Autodesk Inventor part; units mm, degrees
ref_plane "Work Plane1" through (36.5, 52.55, -8.75) normal (0, 0, 1) x (1, 0, 0)
ref_plane "YZ Plane" through (0, 0, 0) normal (1, 0, 0) x (0, 1, 0)
ref_plane "XZ Plane" through (0, 0, 0) normal (0, 1, 0) x (-1, 0, 0)
sketch "Sketch1" plane through (0, 0, 0) normal (0, 0, 1) x (1, 0, 0)
  line L0 (0, 44.8) -> (0, 9.25)
  line L1 (0, 44.8) -> (40, 44.8)
  line L2 (0, 9.25) -> (40, 9.25)
  line L3 (40, 9.25) -> (40, 44.8)
  line L4 (14.9707, 35.95) -> (34.6293, 35.95)
  line L5 (34.6293, 35.95) -> (34.6293, 40.05)
  line L6 (34.6293, 40.05) -> (14.9707, 40.05)
  line L7 (14.9707, 40.05) -> (14.9707, 35.95)
  line L8 (30.8793, 39.05) -> (28.5722, 39.05) construction
  line L9 (30.8793, 39.05) -> (30.8793, 36.95) construction
  line L10 (30.8793, 36.95) -> (28.5722, 36.95) construction
  line L11 (28.5722, 39.05) -> (28.5722, 36.95) construction
  line L12 (30.8793, 39.05) -> (30.8793, 40.05) construction
  line L13 (30.8793, 36.95) -> (30.8793, 35.95) construction
  line L14 (21.0278, 39.05) -> (18.7207, 39.05) construction
  line L15 (21.0278, 39.05) -> (21.0278, 36.95) construction
  line L16 (21.0278, 36.95) -> (18.7207, 36.95) construction
  line L17 (18.7207, 39.05) -> (18.7207, 36.95) construction
  line L18 (18.7207, 39.05) -> (14.9707, 39.05) construction
  line L19 (30.8793, 39.05) -> (34.6293, 39.05) construction
  line L20 (0, -9.25) -> (0, 9.25)
  line L21 (40, 27.025) -> (0, 27.025) construction
  line L22 (14.9707, 18.1) -> (34.6293, 18.1)
  line L23 (34.6293, 18.1) -> (34.6293, 14)
  line L24 (34.6293, 14) -> (14.9707, 14)
  line L25 (14.9707, 14) -> (14.9707, 18.1)
  line L26 (40, 9.25) -> (40, -9.25)
  line L27 (40, -9.25) -> (0, -9.25)
  line L28 (32.375, -9.25) -> (32.375, 9.25)
  line L29 (36.5, 9.25) -> (36.5, -9.3)
  line L30 (0, 44.8) -> (40, 44.8)
  line L31 (0, 63.3) -> (0, 44.8)
  line L32 (40, 44.8) -> (40, 63.3)
  line L33 (40, 63.3) -> (0, 63.3)
  line L34 (32.375, 63.3) -> (32.375, 44.8)
  line L35 (36.5, 44.8) -> (36.5, 63.35)
  point P0 (36.5, -9.25)
  point P1 (36.5, 63.3)
  dimension "d1" = 35.55
  dimension "d2" = 1
  dimension "d3" = 3.75
  dimension "d4" = 40
extrude "Extrusion1" add sketch "Sketch1" along normal blind 2.75
ref_plane "Work Plane1" through (36.5, 52.55, -8.75) normal (0, 0, 1) x (1, 0, 0)
extrude "Extrusion2" add sketch "Sketch1" against normal up to surface (8.75 mm away) contours L35 L33 L32 L1 | L2 L26 L27 L29
ref_plane "Work Plane2" through (27.7797, 32.4377, -8.357) normal (-0.3827, 0, -0.9239) x (-0.4619, -0.866, 0.1913)
sketch "Sketch3" plane through (27.7797, 32.4377, -8.357) normal (-0.3827, 0, -0.9239) x (-0.4619, -0.866, 0.1913)
  circle A0 centre (5.5343, -1.2396) radius 6.25 construction
  ellipse E0 centre (5.5343, -1.2396) end of major axis (-0.7444, 2.3854) minor radius 7.25
  line L0 (10.947, -4.3646) -> (11.813, -4.8646) construction
  line L1 (2.4093, -6.6522) -> (1.9093, -7.5183) construction
  line L2 (0.6415, -9.7142) -> (19.1191, 22.2899) construction
  point P0 (42.5234, 8.7774)
  dimension "d9" = 1
extrude "Extrusion3" cut sketch "Sketch3" against normal blind 17.75
properties part number "Encoderadapter"
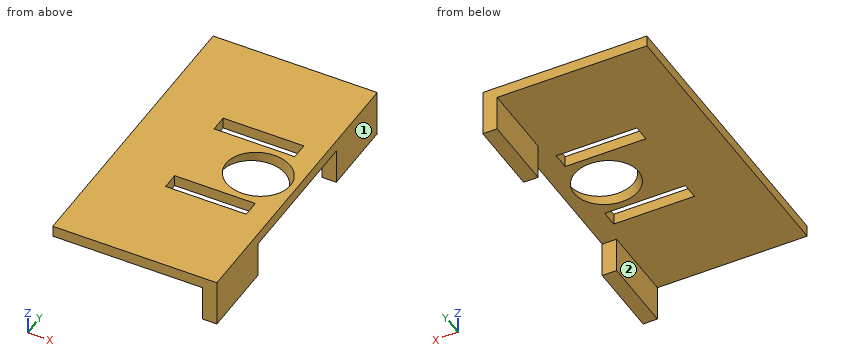
Read the model definition and answer for the solid it produces. Units are mm, in the model's axes. Face numbers are marked on the shaded views. A direction names the side the tool comes from. Give positions to 0.01 mm unless a question says otherwise; leave off trailing zeros. Order: outer loops, then holes, each group sorted by start corner. A loop starts at its lowest first (then second) coordinate and runs counter-clockwise, first axis right, second up. Notation, with made-up numbers: (81.5, -7) -> (134.5, -7) arc R18 ccw to (134.5, 26) -> close; hole circle Ø2 at (28.5, 89). An arc over 180 degrees is marked (long way). One line per item, written item: value. Start each with the question number.
(1) Flat-ended cylindrical pins translate along their axes: P1, Ø10, axis at x = 30.5, y = 26, coming from the +Z side; P2, Ø5, axis at y = 9, z = -3, coming from the -X side; P3, Ø1.5, axis at x = 28.5, y = 36, coming from the -Z side. Find the tip coordinate at first contact, or state that the pin passes through.
(2) The part is cut by section C-C (y = -3). Determine the outline of the cut face in (x, z).
(3) The part is cut by section A-A (z = -3.5). Determine the outline of the cut face in (x, y).
(4) The part is cut by section D-D (x = 4). Determine the outline of the cut face in (y, z).
(5) The part is cut by section B-B (x = 16). Determine the outline of the cut face in (y, z), and give its area (3 significant figures).
(6) Straight lines are drawn through the part: L1, parallel to Y at x = 38, z = -3; L2, parallel to Z at x = 31, y = 7.5; L3, parallel to X at y = 3, z = -7.25. For each, find the intervals that lie inside material, in ascending order.
(7) A tool of negligible diameter and unlimited length cuts with its end or side. For the marked faces 1 and 2, from which of +Z, -Z, +X, -X, +Y, -Y can it reach the whole face along a straight path? Write none if from no direction.
Taken from the geometry:
1. P1: through
1. P2: x = 36.5
1. P3: z = 0
2. outline: (0, 0) -> (36.5, 0) -> (36.5, -8.75) -> (40, -8.75) -> (40, 2.75) -> (0, 2.75) -> close
3. outline: (36.5, -9.25) -> (40, -9.25) -> (40, 9.25) -> (36.5, 9.25) -> close; (36.5, 44.8) -> (40, 44.8) -> (40, 63.3) -> (36.5, 63.3) -> close
4. outline: (-9.25, 0) -> (63.3, 0) -> (63.3, 2.75) -> (-9.25, 2.75) -> close
5. outline: (-9.25, 0) -> (14, 0) -> (14, 2.75) -> (-9.25, 2.75) -> close; (18.1, 0) -> (35.95, 0) -> (35.95, 2.75) -> (18.1, 2.75) -> close; (40.05, 0) -> (63.3, 0) -> (63.3, 2.75) -> (40.05, 2.75) -> close
5. area: 177 mm^2
6. L1: -9.25 to 9.25, 44.8 to 63.3
6. L2: 0 to 2.75
6. L3: 36.5 to 40
7. face 1: +Z, -Z, +X, +Y, -Y
7. face 2: -Z, -X, +Y, -Y
